Autodesk Inventor part; units mm, degrees
ref_plane "YZ Plane" through (0, 0, 0) normal (1, 0, 0) x (0, 1, 0)
ref_plane "XZ Plane" through (0, 0, 0) normal (0, 1, 0) x (-1, 0, 0)
ref_plane "XY Plane" through (0, 0, 0) normal (0, 0, 1) x (1, 0, 0)
sketch "Skizze1" plane through (0, 0, 0) normal (0, 0, 1) x (1, 0, 0)
  line L0 (-89, -12) -> (89, -12)
  line L1 (89, -12) -> (89, 12)
  line L2 (89, 12) -> (-89, 12)
  line L3 (-89, 12) -> (-89, -12)
  line L4 (-89, -12) -> (89, 12) construction
  line L5 (89, -12) -> (-89, 12) construction
  line L6 (65, 12) -> (65, -12)
  line L7 (-65, 12) -> (-65, -12)
  line L8 (-89, 12) -> (-65, -12) construction
  line L9 (-65, 12) -> (-89, -12) construction
  line L10 (89, 12) -> (65, -12) construction
  line L11 (65, 12) -> (89, -12) construction
  point P0 (0, 0)
  dimension "d0" = 178
  dimension "d1" = 24
  dimension "d2" = 24
  dimension "d3" = 24
extrude "Extrusion1" add sketch "Skizze1" along normal blind 5
sketch "Skizze3" plane through (0, 0, 5) normal (0, 0, 1) x (1, 0, 0)
  line L0 (-89, -12) -> (89, -12)
  line L1 (89, -12) -> (89, 12)
  line L2 (89, 12) -> (-89, 12)
  line L3 (-89, 12) -> (-89, -12)
  line L4 (-89, -12) -> (89, 12) construction
  line L5 (89, -12) -> (-89, 12) construction
  line L6 (65, 12) -> (65, -12)
  line L7 (-65, 12) -> (-65, -12)
  line L8 (-89, 12) -> (-65, -12) construction
  line L9 (-65, 12) -> (-89, -12) construction
  line L10 (89, 12) -> (65, -12) construction
  line L11 (65, 12) -> (89, -12) construction
  line L12 (70.15, -6.85) -> (83.85, -6.85)
  line L13 (83.85, -6.85) -> (83.85, 6.85)
  line L14 (83.85, 6.85) -> (70.15, 6.85)
  line L15 (70.15, 6.85) -> (70.15, -6.85)
  line L16 (70.15, -6.85) -> (83.85, 6.85) construction
  line L17 (83.85, -6.85) -> (70.15, 6.85) construction
  line L18 (-83.85, -6.85) -> (-70.15, -6.85)
  line L19 (-70.15, -6.85) -> (-70.15, 6.85)
  line L20 (-70.15, 6.85) -> (-83.85, 6.85)
  line L21 (-83.85, 6.85) -> (-83.85, -6.85)
  line L22 (-83.85, -6.85) -> (-70.15, 6.85) construction
  line L23 (-70.15, -6.85) -> (-83.85, 6.85) construction
  point P0 (0, 0)
  point P1 (0, 0)
  point P2 (77, 0)
  point P3 (-77, 0)
  dimension "d10" = 178
  dimension "d11" = 24
  dimension "d12" = 24
  dimension "d13" = 24
  dimension "d14" = 13.7
  dimension "d15" = 13.7
extrude "Extrusion2" add sketch "Skizze3" along normal blind 2.85 contours L15 L14 L13 L12 | L21 L20 L19 L18
sketch "Skizze4" plane through (0, 0, 0) normal (0, 0, -1) x (-1, 0, 0)
  line L0 (-89, -12) -> (89, -12)
  line L1 (89, -12) -> (89, 12)
  line L2 (89, 12) -> (-89, 12)
  line L3 (-89, 12) -> (-89, -12)
  line L4 (-89, -12) -> (89, 12) construction
  line L5 (89, -12) -> (-89, 12) construction
  line L6 (65, 12) -> (65, -12)
  line L7 (-65, 12) -> (-65, -12)
  line L8 (-89, 12) -> (-65, -12) construction
  line L9 (-65, 12) -> (-89, -12) construction
  line L10 (89, 12) -> (65, -12) construction
  line L11 (65, 12) -> (89, -12) construction
  line L12 (70, -7) -> (84, -7)
  line L13 (84, -7) -> (84, 7)
  line L14 (84, 7) -> (70, 7)
  line L15 (70, 7) -> (70, -7)
  line L16 (70, -7) -> (84, 7) construction
  line L17 (84, -7) -> (70, 7) construction
  line L18 (-84, -7) -> (-70, -7)
  line L19 (-70, -7) -> (-70, 7)
  line L20 (-70, 7) -> (-84, 7)
  line L21 (-84, 7) -> (-84, -7)
  line L22 (-84, -7) -> (-70, 7) construction
  line L23 (-70, -7) -> (-84, 7) construction
  point P0 (0, 0)
  point P1 (0, 0)
  point P2 (0, 0)
  point P3 (77, 0)
  point P4 (-77, 0)
  dimension "d18" = 178
  dimension "d19" = 24
  dimension "d20" = 24
  dimension "d21" = 24
  dimension "d22" = 14
  dimension "d23" = 14
extrude "Extrusion3" cut sketch "Skizze4" against normal blind 3 contours L15 L14 L13 L12 | L21 L20 L19 L18
properties part number "20210330_Stabilisator_Korpus" material "Acetal Resin, Black"
Model file for the job. Use its own axes, mm. A direction names the side the tool comes from. Coordinates: 2 decimals unless noted, no trailing zeros. Write each loop counter-clockwise with the first axis right and the second up, starting at its lowest first coordinate (ties: lowest second). Pieces come first, ordered by that corner, then holes. Notation, with made-up numbers: (-35, 62.25) - (-25, 62.25) arc R18 ccw to (-25, 86.25) - close; hole circle Ø8 at (24, -9). An arc over 180 degrees is marked (long way). Write each question's results on one line, items separated by ' | '. Start each with the question number.
1) Cut at C-C (y = 1.25). Write the cut outline in (x, z).
2) Cut at D-D (x = 40). Write the cut outline in (y, z).
3) Probe line 1 along X through (y, z) = (4, 2.25); line 2 along Y through (x, z) = (-80, 1); line 3 along X through (y, z) = (2.25, 6). List the from-to ranges inside material, lowest first. Write a range as from..to.
4) Flat gauge pins, fed straight in: P1, Ø2.5, axis at y = 1.5, z = 6.5, coming from the +X side; P2, Ø8, axis at x = -11, y = 6.5, coming from the +Z side; P3, Ø2.5, axis at x = 76, z = 7, coming from the -Y side; P4, Ø4, axis at y = -7.5, z = 6.5, coming from the -X side. Where does each tip first touch, or does it go through?
5) Cut at B-B (x = -77.5). Write the cut outline in (y, z), then the cut area to 3 significant figures.
6) Cut at A-A (z = 6.25). Write the cut outline in (x, y).
7) Mould opens along Y. For faces 1 (the face through (70, 0, 1)), 2 (the face through (-77, 6.85, 6)), 3 (the face through (70.15, 0, 6)), 4 (the face through (-77, -6.85, 6)) say: pulls with the +Y half, pulls with the -Y half, needs draft (parallel to the pull), parting line crosses it, or undercut.
8) 3-axis set-ups, long thin cutter, end or side, ignore diameter. For faces 5 (the face through (77, -6.85, 6)), 6 (the face through (77, -7, 1)), 7 (the face through (-70.15, 0, 6)): which of +Z, -Z, +X, -X, +Y, -Y reach the whole face in a straight line?
Returned:
1) outline: (-89, 0) - (-84, 0) - (-84, 3) - (-70, 3) - (-70, 0) - (70, 0) - (70, 3) - (84, 3) - (84, 0) - (89, 0) - (89, 5) - (83.85, 5) - (83.85, 7.85) - (70.15, 7.85) - (70.15, 5) - (-70.15, 5) - (-70.15, 7.85) - (-83.85, 7.85) - (-83.85, 5) - (-89, 5) - close
2) outline: (-12, 0) - (12, 0) - (12, 5) - (-12, 5) - close
3) line 1: -89..-84, -70..70, 84..89 | line 2: -12..-7, 7..12 | line 3: -83.85..-70.15, 70.15..83.85
4) P1: x = 83.85 | P2: z = 5 | P3: y = -6.85 | P4: x = -89
5) outline: (-12, 0) - (-7, 0) - (-7, 3) - (7, 3) - (7, 0) - (12, 0) - (12, 5) - (6.85, 5) - (6.85, 7.85) - (-6.85, 7.85) - (-6.85, 5) - (-12, 5) - close | area: 117 mm^2
6) outline: (-83.85, -6.85) - (-70.15, -6.85) - (-70.15, 6.85) - (-83.85, 6.85) - close; (70.15, -6.85) - (83.85, -6.85) - (83.85, 6.85) - (70.15, 6.85) - close
7) face 1: undercut | face 2: pulls with the +Y half | face 3: needs draft | face 4: pulls with the -Y half
8) face 5: +Z, +X, -X, -Y | face 6: -Z | face 7: +Z, +Y, -Y
